Design review of the part built by this model. Coordinates are the model's own, in mm. A direction names the side the tool comes from. Coordinates: 2 decimals unless noted, no trailing zeros. Loops run counter-clockwise (first coordinate to the right, second up) from the corner with the lowest first, then second, coordinate; pieces in that order, holes last. Notation, with made-up numbers: (-32, -15) -> (-28, -15) arc R26 cw to (-28, 14) -> close; hole circle Ø8 at (-8.75, 17.25). An arc over 180 degrees is marked (long way). One line per item, written item: value. Start each with the question number.
1. Insertion check: pin 1 (2 mm diameter, centred on x = 59, y = -9, fed in from -Z). The pin has a flat end and moves straight along its axis. Give the tip position at first contact, or say it passes through.
2. Add section C-C on x = 0. Write out the cut boundary in (y, z) (3 decimals), plus the area to 3 significant figures.
3. Machinability: for faces 4 (the flat face through (0, -44.45, 6)), 5 (the flat face through (-38.1, -1, -6)), 6 (the flat face through (-57, 1, 0)), which of the approach directions +Z, -Z, +X, -X, +Y, -Y give a long, thin tool a straight path to every point of the face, cutting with its end or side? Answer none if there is none.
4. Add section A-A on z = -4.5. Write out the cut boundary in (x, y).
5. Add section B-B on y = 4. Write out the cut boundary in (x, z), plus the area to 3 significant figures.
6. Draft analysis for pull direction X (two halves, no side actions). For faces 1 (the flat face through (76.2, -1, 0)), 2 (the flat face through (-45, -1, -12.7)), 3 (the cylindrical face through (1.707, -50.889, 9.027)), state which applies: pulls with the +X half, pulls with the -X half, needs draft (parallel to the pull), parting line crosses it, or undercut.
7. For probe 1 along Z at (x, y) = (0, -49.75) (3 decimals); probe 2 along X at (y, z) = (19.5, -5.5); probe 3 along X at (y, z) = (24, -3), list the stretches that pass through material, from the lowest coordinate up.
```python
from build123d import *

# Parameters (mm, degrees)
F0_W     = 152.4
F0_H     = 114.3
F1_DEPTH = 12.7
F2_W     = 6.35
F2_H     = 12.7
F3_DEPTH = 114.3
F4_R     = 3.175
F5_DEPTH = 12.7


with BuildPart() as f1:
    # F0 (on Top) → F1 (new body)
    with BuildSketch(Plane.XY):
        Rectangle(F0_W, F0_H)
    extrude(amount=F1_DEPTH)

    # F2 (on face) → F3 (join)
    with BuildSketch(Plane.XZ.offset(57.15)):
        Polygon((-63.5, -12.7), (-69.85, 0), (-69.85, -12.7), align=None)
        with Locations((-73.025, -6.35)):
            Rectangle(F2_W, F2_H)
        Polygon((-44.45, -12.7), (-44.45, 0), (-50.8, -12.7), align=None)
        with Locations((-41.275, -6.35)):
            Rectangle(F2_W, F2_H)
        with Locations((41.275, -6.35)):
            Rectangle(F2_W, F2_H)
        Polygon((50.8, -12.7), (44.45, 0), (44.45, -12.7), align=None)
        Polygon((69.85, -12.7), (69.85, 0), (63.5, -12.7), align=None)
        with Locations((73.025, -6.35)):
            Rectangle(F2_W, F2_H)
    extrude(amount=-F3_DEPTH)

    # F4 (on face) → F5 (cut)
    with BuildSketch(Plane.XZ.offset(57.15)):
        with Locations((0, 6.35)):
            Circle(F4_R)
    extrude(amount=-F5_DEPTH, mode=Mode.SUBTRACT)


solid = f1.part
```
Worked answers:
1. pin 1: stops at z = 0
2. outline: (-57.15, 0) -> (57.15, 0) -> (57.15, 12.7) -> (-57.15, 12.7) -> (-57.15, 9.525) -> (-44.45, 9.525) -> (-44.45, 3.175) -> (-57.15, 3.175) -> close
2. area: 1,370 mm²
3. face 4: -Y
3. face 5: -Z, +Y, -Y
3. face 6: +Y, -Y
4. outline: (-76.2, -57.15) -> (-67.6, -57.15) -> (-67.6, 57.15) -> (-76.2, 57.15) -> close; (-46.7, -57.15) -> (-38.1, -57.15) -> (-38.1, 57.15) -> (-46.7, 57.15) -> close; (38.1, -57.15) -> (46.7, -57.15) -> (46.7, 57.15) -> (38.1, 57.15) -> close; (67.6, -57.15) -> (76.2, -57.15) -> (76.2, 57.15) -> (67.6, 57.15) -> close
5. outline: (-76.2, -12.7) -> (-63.5, -12.7) -> (-69.85, 0) -> (-44.45, 0) -> (-50.8, -12.7) -> (-38.1, -12.7) -> (-38.1, 0) -> (38.1, 0) -> (38.1, -12.7) -> (50.8, -12.7) -> (44.45, 0) -> (69.85, 0) -> (63.5, -12.7) -> (76.2, -12.7) -> (76.2, 12.7) -> (-76.2, 12.7) -> close
5. area: 2,420 mm²
6. face 1: pulls with the +X half
6. face 2: needs draft
6. face 3: undercut
7. probe 1: z = 0 to 3.175, 9.525 to 12.7
7. probe 2: x = -76.2 to -67.1, -47.2 to -38.1, 38.1 to 47.2, 67.1 to 76.2
7. probe 3: x = -76.2 to -68.35, -45.95 to -38.1, 38.1 to 45.95, 68.35 to 76.2
